Verification items for the finished model (mm, model axes). A direction names the side the tool comes from. Coordinates: 2 decimals unless noted, no trailing zeros. Order: outer loops, then holes, each group sorted by start corner. A loop starts at its lowest first (then second) coordinate and runs counter-clockwise, first axis right, second up. Notation, with made-up numbers: M -25.5,70 L 2.5,70 A31 ccw 2.5,98 Z; hole C 27,62 d4. An arc over 180 degrees is marked long. Return JSON: item names as keys, results as strings. Group by question number.
1. Mould release check, pull along Y, two halves, no side actions. Record for faces 4 (the flat face through (1, 0, 1.588)), 5 (the cylindrical face through (32.57, -20.79, 0.81)), 6 (the flat face through (0, 26.67, 1)): +Y half, -Y half, draft (parallel to the pull), parting line (faces both ways), or undercut.
2. Gauge pin test, flat end, axial feed: pin 1 (0.8 mm diameter, centred on y = 19.5, z = 0.5, fed in from +X). Record the tip position at first contact, or that the pin passes through.
3. Set-up check for faces 1 (the flat face through (33.02, 20, 1)), 2 (the flat face through (33.02, -25, 1)), 3 (the cylindrical face through (-17.12, 22.52, 0.81)): record each of +Z, -Z, +X, -X, +Y, -Y from which the full face is reachable in a straight line by a thin tool's end or side.
4. Section check A-A, the plane z = 1.25. Record the cut outline in (x, y) (1 decimal), plus the area to 3 significant figures.
5. Material ranges on line 1 along X through (y, z) = (-19, 0.85); line 2 along X through (y, z) = (14.5, 1); line 3 along X through (y, z) = (8, 1.2), recorded low to high.
```python
from build123d import *

# Parameters (mm, degrees)
F1_DEPTH = 1.588
F2_R     = 1.6195
F3_DEPTH = 1.589


with BuildPart() as f1:
    # F0 (on Top) → F1 (new body)
    with BuildSketch(Plane.XY):
        Polygon((33.02, 26.67), (-33.02, 26.67), (-33.02, -26.67), (33.02, -26.67), (33.02, -24.003), (35.56, -21.463), (35.56, 11.557), (33.02, 14.097), align=None)
    extrude(amount=F1_DEPTH)

    # F2 (on face) → F3 (cut, through all)
    with BuildSketch(Plane.XY.offset(1.588)):
        with Locations((-17.863, 23.959)):
            Circle(F2_R)
        with Locations((-19.006, -23.959)):
            Circle(F2_R)
        with Locations((32.925, 8.719)):
            Circle(F2_R)
        with Locations((32.925, -19.209)):
            Circle(F2_R)
    extrude(amount=-F3_DEPTH, mode=Mode.SUBTRACT)


solid = f1.part
```
Answers follow:
{
 "1": {"face 4": "draft", "face 5": "undercut", "face 6": "+Y half"},
 "2": {"pin 1": "x = 33.02"},
 "3": {"face 1": "+Z, -Z, +X, +Y", "face 2": "+Z, -Z, +X, -Y", "face 3": "+Z, -Z"},
 "4": {"outline": "M -33,-26.7 L 33,-26.7 L 33,-24 L 35.6,-21.5 L 35.6,11.6 L 33,14.1 L 33,26.7 L -33,26.7 Z; hole C -19,-24 d3.2; hole C -17.9,24 d3.2; hole C 32.9,-19.2 d3.2; hole C 32.9,8.7 d3.2", "area": "3,580 mm^2"},
 "5": {"line 1": "-33.02 to 31.32, 34.53 to 35.56", "line 2": "-33.02 to 33.02", "line 3": "-33.02 to 31.47, 34.38 to 35.56"}
}
